Verification items for the finished model (mm, model axes). A direction names the side the tool comes from. Coordinates: 2 decimals unless noted, no trailing zeros. Order: outer loops, then holes, each group sorted by start corner. A loop starts at its lowest first (then second) coordinate and runs counter-clockwise, first axis right, second up. Notation, with made-up numbers: (4.25, 6) -> (36.25, 6) arc R34 cw to (36.25, 37) -> close; hole circle Ø9 at (-31.75, 31). An arc over 180 degrees is marked (long way). Write item = value, one per line. Start each with the question number.
1. Cross-section at A-A on y = -52. Record the cut outline in (x, z).
2. Thickness scan on line 1 along X through (y, z) = (-94, -27.5); line 2 along Y through (x, z) = (-839.25, 0); line 3 along X through (y, z) = (12.5, 0). Record the ranges inside material, lowest first. Write a range as from..to.
3. Release check for a two-part mould opening along X. For faces 1 (the flat face through (11, 2.537, -27)), 2 (the flat face through (-846, -80, 1)), 3 (the flat face through (4, 18, 63)) record: +X half, -X half, draft (parallel to the pull), parting line (faces both ways), or undercut.
4. Cross-section at B-B on x = 261. Record the cut outline in (y, z).
5. Set-up check for faces 4 (the flat face through (4, 18, -63)), 5 (the flat face through (819, -72, 1)), 6 (the cylindrical face through (21.77, 31.82, -34.15)): record each of +Z, -Z, +X, -X, +Y, -Y from which the full face is reachable in a straight line by a thin tool's end or side.
6. Go/stop test with flat-tipped pins: P1, Ø1, axis at x = -206, z = -38, coming from the -Y side; P2, Ø1, axis at x = 311.5, z = 37.5, coming from the +Y side. Record where each tip stops, or that it passes through.
from build123d import *

# Parameters (mm, degrees)
BOSS_EXTRUDE1_DEPTH     = 3.5
CUT_EXTRUDE1_DEPTH      = 49.633835958
CUT_EXTRUDE1_DEPTH_BACK = 1.5
SKETCH2_R               = 1.25
SKETCH3_R               = 2.25
SKETCH3_R_2             = 1.25
BOSS_EXTRUDE2_DEPTH     = 0.25
CUT_EXTRUDE2_DEPTH      = 49.633835958
CUT_EXTRUDE2_DEPTH_BACK = 49.633835958
SKETCH4_R               = 1.5
SCALE1_SCALE            = 18


with BuildPart() as part:
    # Sketch1 → Boss-Extrude1 (new, symmetric)
    with BuildSketch(Plane.XY):
        Polygon((-47, -12), (-47, 0), (47, 0), (47, -12), (45.5, -12), (45.5, -1.5), (-45.5, -1.5), (-45.5, -12), align=None)
    extrude(amount=BOSS_EXTRUDE1_DEPTH, both=True)

    # Sketch2 → Cut-Extrude1 (cut, two sides: drawn at the far end of the back side and taken through both)
    with BuildSketch(Plane(origin=(0, 0, 0), x_dir=(1, 0, 0), z_dir=(0, 1, 0)).offset(-CUT_EXTRUDE1_DEPTH_BACK)):
        with Locations(Location((0, 0, 0), (0, 0, 270))):
            Circle(SKETCH2_R)
    extrude(amount=CUT_EXTRUDE1_DEPTH + CUT_EXTRUDE1_DEPTH_BACK, mode=Mode.SUBTRACT)

    # Sketch3 → Boss-Extrude2 (add, symmetric)
    with BuildSketch(Plane(origin=(0, 0, 0), x_dir=(1, 0, 0), z_dir=(0, 1, 0))):
        Circle(SKETCH3_R)
        with Locations(Location((0, 0, 0), (0, 0, 180))):
            Circle(SKETCH3_R_2, mode=Mode.SUBTRACT)
    extrude(amount=BOSS_EXTRUDE2_DEPTH, both=True)

    # Sketch4 → Cut-Extrude2 (cut, two sides: drawn at the far end of the back side and taken through both)
    with BuildSketch(Plane(origin=(0, 0, 0), x_dir=(0, 0, -1), z_dir=(1, 0, 0)).offset(-CUT_EXTRUDE2_DEPTH_BACK)):
        with Locations((0, -8)):
            Circle(SKETCH4_R)
    extrude(amount=CUT_EXTRUDE2_DEPTH + CUT_EXTRUDE2_DEPTH_BACK, mode=Mode.SUBTRACT)


with BuildPart() as part_1:
    # Scale1: scaled about (0, -1.737452604, 0)
    add(part.part.scale(SCALE1_SCALE).moved(Location((0, 29.536694268, 0))))


solid = part_1.part
Worked out:
q1.outline = (-846, -63) -> (-819, -63) -> (-819, 63) -> (-846, 63) -> close; (819, -63) -> (846, -63) -> (846, 63) -> (819, 63) -> close
q2.line_1 = -846..-819, 819..846
q2.line_2 = -186.46..-141.46, -87.46..29.54
q2.line_3 = -846..-22.5, 22.5..846
q3.face_1 = undercut
q3.face_2 = -X half
q3.face_3 = draft
q4.outline = (2.54, -63) -> (29.54, -63) -> (29.54, 63) -> (2.54, 63) -> close
q5.face_4 = -Z, +X, -X, +Y, -Y
q5.face_5 = +Z, -Z, -Y
q5.face_6 = +Y
q6.P1 = 2.54
q6.P2 = 29.54
